CAD build for the part. Positions are in the model's coordinates, mm. A direction names the side the tool comes from. Coordinates: 2 decimals unless noted, no trailing zeros. Loops run counter-clockwise (first coordinate to the right, second up) from the corner with the lowest first, then second, coordinate; pieces in that order, holes last. Notation, with made-up numbers: (19, -17.75) -> (27, -17.75) arc R13 ccw to (27, -11.75) -> close; hole circle Ø9 at (9, 38.5). An arc over 180 degrees is marked (long way). Write each question's results on one line, items separated by ' | '.
from build123d import *

# Parameters (mm, degrees)
F0_W     = 25.4
F0_H     = 247.304687
F0_R     = 10.16
F1_DEPTH = 12.7
F2_DEPTH = 25.4


with BuildPart() as f1:
    # F0 (on Front) → F1 (new body)
    with BuildSketch(Plane.XZ):
        with Locations((12.7, -23.54492)):
            Rectangle(F0_W, F0_H)
        with Locations((13.056295, -14.342986)):
            Circle(F0_R, mode=Mode.SUBTRACT)
    extrude(amount=F1_DEPTH)

    # F0 (on Front) → F2 (join)
    with BuildSketch(Plane.XZ):
        with Locations((13.056295, -14.342986)):
            Circle(F0_R)
    extrude(amount=F2_DEPTH)


solid = f1.part
1) Which spindle directions (+Z, -Z, +X, -X, +Y, -Y) get a long thin tool onto all of the face, cutting with end or side? Do faces 1 (the cylindrical face through (10.85, -18.96, -24.26)), 2 (the flat face through (13, -25.4, -14)). Say none if no direction does.
Outcome:
face 1: -Y | face 2: +Z, -Z, +X, -X, -Y
2) Slice it at A-A (x = 21). Write the cut outline in (y, z).
Outcome:
outline: (-25.4, -20.68) -> (-12.7, -20.68) -> (-12.7, -147.2) -> (0, -147.2) -> (0, 100.11) -> (-12.7, 100.11) -> (-12.7, -8.01) -> (-25.4, -8.01) -> close
3) Pin check, flat tips, straight feed: pin 1 (10 mm diameter, centred on y = -13.5, z = 40, fed in from +X); pin 2 (4 mm diameter, centred on x = 19, y = -20, fed in from +Z); pin 3 (2 mm diameter, centred on x = 16, z = -108, fed in from -Y). Stop position of each tip, or through.
Outcome:
pin 1: stops at x = 25.4 | pin 2: stops at z = -4.98 | pin 3: stops at y = -12.7
4) Slice it at D-D (x = 6). Write the cut outline in (y, z).
Outcome:
outline: (-25.4, -21.65) -> (-12.7, -21.65) -> (-12.7, -147.2) -> (0, -147.2) -> (0, 100.11) -> (-12.7, 100.11) -> (-12.7, -7.03) -> (-25.4, -7.03) -> close
5) Slice it at B-B (z = 29.5). Write the cut outline in (x, y), then the cut area to 3 significant figures.
Outcome:
outline: (0, -12.7) -> (25.4, -12.7) -> (25.4, 0) -> (0, 0) -> close | area: 323 mm^2
6) Slice it at C-C (y = -17.5). Write the cut outline in (x, z).
Outcome:
outline: circle Ø20.32 at (13.06, -14.34)
7) Drill centre lines: L1, parallel to Y at x = 15.5, z = 16; L2, parallel to Z at x = 13.75, y = -23; L3, parallel to Z at x = 9.75, y = -13.5. Where is each one in solid material? Low to high. Write a range as from..to.
Outcome:
L1: y = -12.7..0 | L2: z = -24.48..-4.21 | L3: z = -23.95..-4.74
